```python
from build123d import *

# Parameters (mm, degrees)
SKETCH1_W                    = 2220
SKETCH1_H                    = 969
BASE_FLANGE1_DEPTH           = 4
EDGE_FLANGE1_START           = -788.522727273
EDGE_FLANGE1_DEPTH           = 2220
EDGE_FLANGE1_2_DEPTH         = 2220
EDGE_FLANGE2_START           = -788.522727273
EDGE_FLANGE2_DEPTH           = 2220
EDGE_FLANGE2_2_DEPTH         = 2220
EDGE_FLANGE3_STRIP_W         = 24
EDGE_FLANGE3_STRIP_H         = 4
EDGE_FLANGE3_STRIP_CUT_DEPTH = 954.890119211
EDGE_FLANGE3_DEPTH           = 954.890119211
EDGE_FLANGE4_STRIP_W         = 24
EDGE_FLANGE4_STRIP_H         = 4
EDGE_FLANGE4_STRIP_CUT_DEPTH = 954.890119211
EDGE_FLANGE4_DEPTH           = 954.890119211
CUT_EXTRUDE1_DEPTH           = 1665.285512579
LPATTERN1_COUNT              = 7
LPATTERN1_PITCH              = 300
CUT_EXTRUDE2_DEPTH           = 1665.285512579
CUT_EXTRUDE2_DEPTH_BACK      = 1665.285512579
SKETCH20_R                   = 7
CUT_EXTRUDE3_DEPTH           = 2327.408738422
LPATTERN2_COUNT              = 5
LPATTERN2_PITCH              = 190
CUT_EXTRUDE4_DEPTH           = 1704.883654617
LPATTERN3_COUNT              = 7
LPATTERN3_PITCH              = 300


# Read off the part's stored shape, not the designer's step: Edge-Flange1, Edge-Flange2
# Sheet-metal steps are written as plain solids
with BuildPart() as part:
    # Sketch1 → Base-Flange1 (new body)
    with BuildSketch(Plane(origin=(0, 0, 0), x_dir=(0, 0, -1), z_dir=(1, 0, 0))):
        with Locations((-321.477272727, 132.136363636)):
            Rectangle(SKETCH1_W, SKETCH1_H)
    extrude(amount=-BASE_FLANGE1_DEPTH)

    # Edge-Flange1 outline → Edge-Flange1 (cut)
    with BuildSketch(Plane.XY.offset(EDGE_FLANGE1_START)):
        with BuildLine():
            Line((-4, 616.636363636), (-2.965436872, 615.798590934))
            ThreePointArc((-2.965436872, 615.798590934), (-0.779317725, 613.025512017), (0, 609.581423242))
            Line((0, 609.581423242), (0, 616.636363636))
            Line((0, 616.636363636), (-4, 616.636363636))
        make_face()
    extrude(amount=EDGE_FLANGE1_DEPTH, mode=Mode.SUBTRACT)

    # Edge-Flange1 2 outline → Edge-Flange1 2 (add)
    with BuildSketch(Plane.XY.offset(EDGE_FLANGE1_START)):
        with BuildLine():
            Line((-4, 609.581423242), (-4, 616.636363636))
            Line((-4, 616.636363636), (-93.257515375, 688.91567443))
            Line((-93.257515375, 688.91567443), (-95.774796939, 685.807090584))
            Line((-95.774796939, 685.807090584), (-5.482718436, 612.690007088))
            ThreePointArc((-5.482718436, 612.690007088), (-4.389658863, 611.303467629), (-4, 609.581423242))
        make_face()
    extrude(amount=EDGE_FLANGE1_2_DEPTH)

    # Edge-Flange2 outline → Edge-Flange2 (cut)
    with BuildSketch(Plane.XY.offset(EDGE_FLANGE2_START)):
        with BuildLine():
            Line((0, -352.363636364), (-1.034563128, -351.525863661))
            ThreePointArc((-1.034563128, -351.525863661), (-3.220682275, -348.752784744), (-4, -345.308695969))
            Line((-4, -345.308695969), (-4, -352.363636364))
            Line((-4, -352.363636364), (0, -352.363636364))
        make_face()
    extrude(amount=EDGE_FLANGE2_DEPTH, mode=Mode.SUBTRACT)

    # Edge-Flange2 2 outline → Edge-Flange2 2 (add)
    with BuildSketch(Plane.XY.offset(EDGE_FLANGE2_START)):
        with BuildLine():
            Line((0, -345.308695969), (0, -352.363636364))
            Line((0, -352.363636364), (34.857298073, -380.590519783))
            Line((34.857298073, -380.590519783), (37.374579637, -377.481935938))
            Line((37.374579637, -377.481935938), (1.482718436, -348.417279815))
            ThreePointArc((1.482718436, -348.417279815), (0.389658863, -347.030740356), (0, -345.308695969))
        make_face()
    extrude(amount=EDGE_FLANGE2_2_DEPTH)

    # Edge-Flange3 strip (across the edge) → Edge-Flange3 strip cut (cut)
    with BuildSketch(Plane(origin=(0, 609.581423242, 1431.477272727), x_dir=(0, 0, -1), z_dir=(0, -1, 0))):
        with Locations((-4, -2)):
            Rectangle(EDGE_FLANGE3_STRIP_W, EDGE_FLANGE3_STRIP_H)
    extrude(amount=EDGE_FLANGE3_STRIP_CUT_DEPTH, mode=Mode.SUBTRACT)

    # Edge-Flange3 section (across the edge) → Edge-Flange3 (add)
    with BuildSketch(Plane(origin=(0, 609.581423242, 1431.477272727), x_dir=(0, 0, -1), z_dir=(0, -1, 0))):
        with BuildLine():
            Line((0, 4), (0, 46))
            Line((0, 46), (4, 46))
            Line((4, 46), (4, 4))
            ThreePointArc((4, 4), (5.171572875, 1.171572875), (8, 0))
            Line((8, 0), (8, -4))
            ThreePointArc((8, -4), (2.343145751, -1.656854249), (0, 4))
        make_face()
    extrude(amount=EDGE_FLANGE3_DEPTH)

    # Edge-Flange4 strip (across the edge) → Edge-Flange4 strip cut (cut)
    with BuildSketch(Plane(origin=(0, -345.308695969, -788.522727273), x_dir=(0, 0, 1), z_dir=(0, 1, 0))):
        with Locations((-4, -2)):
            Rectangle(EDGE_FLANGE4_STRIP_W, EDGE_FLANGE4_STRIP_H)
    extrude(amount=EDGE_FLANGE4_STRIP_CUT_DEPTH, mode=Mode.SUBTRACT)

    # Edge-Flange4 section (across the edge) → Edge-Flange4 (add)
    with BuildSketch(Plane(origin=(0, -345.308695969, -788.522727273), x_dir=(0, 0, 1), z_dir=(0, 1, 0))):
        with BuildLine():
            Line((0, 4), (0, 46))
            Line((0, 46), (4, 46))
            Line((4, 46), (4, 4))
            ThreePointArc((4, 4), (5.171572875, 1.171572875), (8, 0))
            Line((8, 0), (8, -4))
            ThreePointArc((8, -4), (2.343145751, -1.656854249), (0, 4))
        make_face()
    extrude(amount=EDGE_FLANGE4_DEPTH)

    # Sketch18 → Cut-Extrude1 (cut, symmetric)
    with BuildSketch(Plane(origin=(299.99651319, 370.464841108, 0), x_dir=(0.7771459614569677, -0.6293203910498413, 0), z_dir=(0.6293203910498414, 0.7771459614569678, 0))):
        with BuildLine():
            Line((-524.023383081, 943.522727273), (-524.023383081, 933.522727273))
            ThreePointArc((-524.023383081, 933.522727273), (-531.023383081, 926.522727273), (-538.023383081, 933.522727273))
            Line((-538.023383081, 933.522727273), (-538.023383081, 943.522727273))
            ThreePointArc((-538.023383081, 943.522727273), (-531.023383081, 950.522727273), (-524.023383081, 943.522727273))
        make_face()
    cut_extrude1 = extrude(amount=CUT_EXTRUDE1_DEPTH, both=True, mode=Mode.SUBTRACT)

    # LPattern1: Cut-Extrude1 ×7
    with Locations(*[(0, 0, i * LPATTERN1_PITCH) for i in range(1, LPATTERN1_COUNT)]):
        add(cut_extrude1, mode=Mode.SUBTRACT)

    # Sketch19 → Cut-Extrude2 (cut, two sides: drawn at the far end of the back side and taken through both)
    with BuildSketch(Plane(origin=(299.99651319, 370.464841108, 0), x_dir=(0.7771459614569677, -0.6293203910498413, 0), z_dir=(0.6293203910498414, 0.7771459614569678, 0)).offset(-CUT_EXTRUDE2_DEPTH_BACK)):
        with BuildLine():
            Line((484.914799236, -1336.477272727), (484.914799236, -1346.477272727))
            ThreePointArc((484.914799236, -1346.477272727), (477.914799236, -1353.477272727), (470.914799236, -1346.477272727))
            Line((470.914799236, -1346.477272727), (470.914799236, -1336.477272727))
            ThreePointArc((470.914799236, -1336.477272727), (477.914799236, -1329.477272727), (484.914799236, -1336.477272727))
        make_face()
    extrude(amount=CUT_EXTRUDE2_DEPTH + CUT_EXTRUDE2_DEPTH_BACK, mode=Mode.SUBTRACT)

    # Sketch20 → Cut-Extrude3 (cut, symmetric)
    with BuildSketch(Plane.XY.offset(1431.477272727)):
        with Locations((71, -246.525863661)):
            Circle(SKETCH20_R)
    cut_extrude3 = extrude(amount=CUT_EXTRUDE3_DEPTH, both=True, mode=Mode.SUBTRACT)

    # LPattern2: Cut-Extrude3 ×5
    with Locations(*[(0, -i * LPATTERN2_PITCH, 0) for i in range(1, LPATTERN2_COUNT)]):
        add(cut_extrude3, mode=Mode.SUBTRACT)

    # Sketch21 → Cut-Extrude4 (cut, symmetric)
    with BuildSketch(Plane(origin=(-169.814541183, -209.703494046, 0), x_dir=(0.7771459614569678, -0.6293203910498414, 0), z_dir=(0.6293203910498414, 0.7771459614569678, 0))):
        with BuildLine():
            Line((298.602583165, 943.522727273), (298.602583165, 933.522727273))
            ThreePointArc((298.602583165, 933.522727273), (291.602583165, 926.522727273), (284.602583165, 933.522727273))
            Line((284.602583165, 933.522727273), (284.602583165, 943.522727273))
            ThreePointArc((284.602583165, 943.522727273), (291.602583165, 950.522727273), (298.602583165, 943.522727273))
        make_face()
    cut_extrude4 = extrude(amount=CUT_EXTRUDE4_DEPTH, both=True, mode=Mode.SUBTRACT)

    # LPattern3: Cut-Extrude4 ×7
    with Locations(*[(0, 0, i * LPATTERN3_PITCH) for i in range(1, LPATTERN3_COUNT)]):
        add(cut_extrude4, mode=Mode.SUBTRACT)


solid = part.part
```
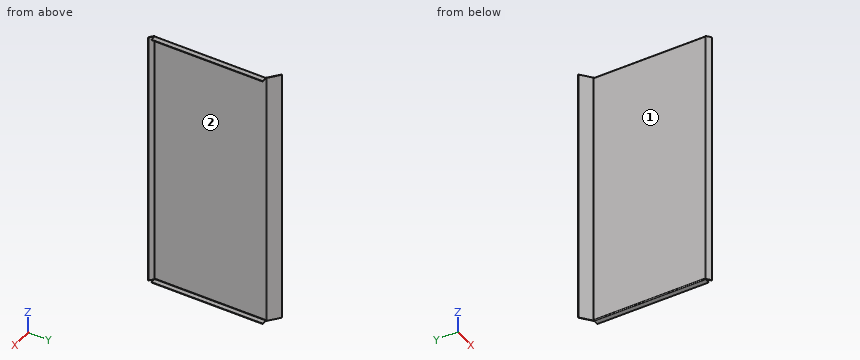
Work out the finished part from the listing and answer in its coordinate system (mm). Face numbers are marked on the shaded views. Give positions to 0.01 mm unless a question says otherwise; leave off trailing zeros. Loops run counter-clockwise (first coordinate to the right, second up) from the corner with the lowest first, then second, coordinate; pieces in that order, holes last. Notation, with made-up numbers: (49, 58.5) -> (65, 58.5) arc R29 ccw to (65, 88.5) -> close; hole circle Ø4 at (45.5, -32.75). An arc over 180 degrees is marked (long way). Put each result on its own line as item: value. Start each with the question number.
Item 1: The part is cut by section A-A (y = -33). Give the vertices of the cut face in (x, z), then the cut area to 3 significant figures.
Item 2: Each of these flat-tipped pins is pushed along its axis until it touches: P1, Ø5, axis at y = 519, z = -229.5, coming from the +X side; P2, Ø4, axis at x = 31, z = 1426.5, coming from the -Y side; P3, Ø5, axis at x = -31.5, z = 119, coming from the +Y side. Where does it stop, or does it pass through?
Item 3: The mould has two halves that part along Z. Classify the marked faces 1 and 2: released by +Z, released by -Z, zero draft, split by the parting line, or undercut.
Item 4: The part is cut by section C-C (x = -45). Give the vertices of the cut face in (y, z).
Item 5: Find the intervals of material crossed by L1, parallel to Z at x = 18, y = 565.5; L2, parallel to X at y = 331.5, z = 114; L3, parallel to Z at x = 3.5, y = 437, in increasing order. Write a range as [from, to].
Item 6: The part is cut by section B-B (z = -608). Give the vertices of the cut face in (x, y), then the cut area to 3 significant figures.
Answers below:
1. outline: (-4, -780.52) arc R8 ccw to (4, -788.52) -> (46, -788.52) -> (46, -784.52) -> (4, -784.52) arc R4 cw to (0, -780.52) -> (0, 1423.48) arc R4 cw to (4, 1427.48) -> (46, 1427.48) -> (46, 1431.48) -> (4, 1431.48) arc R8 ccw to (-4, 1423.48) -> close
1. area: 9,230 mm2
2. P1: x = 0
2. P2: y = -379.09
2. P3: y = 640.93
3. face 1: zero draft
3. face 2: undercut
4. outline: (644.69, -788.52) -> (649.84, -788.52) -> (649.84, 1431.48) -> (644.69, 1431.48) -> close
5. L1: [-788.52, -784.52], [1427.48, 1431.48]
5. L2: [-4, 0]
5. L3: [-788.51, -784.49], [1427.45, 1431.46]
6. outline: (-95.77, 685.81) -> (-5.48, 612.69) arc R4 cw to (-4, 609.58) -> (-4, -345.31) arc R8 ccw to (-1.03, -351.53) -> (34.86, -380.59) -> (37.37, -377.48) -> (1.48, -348.42) arc R4 cw to (0, -345.31) -> (0, 609.58) arc R8 ccw to (-2.97, 615.8) -> (-93.26, 688.92) -> close
6. area: 4,510 mm2
